from build123d import *

# Parameters (mm, degrees)
BOSS_EXTRUDE1_DEPTH = 390.3
BOSS_EXTRUDE2_DEPTH = 4.3
SKETCH3_W           = 8.6
SKETCH3_H           = 70
CUT_EXTRUDE1_DEPTH  = 10
SKETCH4_W           = 230.803227125
SKETCH4_H           = 349.257793427
CUT_EXTRUDE2_DEPTH  = 15


with BuildPart() as part:
    # Sketch1 → Boss-Extrude1 (new body)
    with BuildSketch(Plane.XY):
        Polygon((-30, 0), (-25.7, 0), (-25.7, 20.7), (25.7, 20.7), (25.7, 0), (30, 0), (30, 25), (-30, 25), align=None)
    extrude(amount=BOSS_EXTRUDE1_DEPTH)

    # Sketch2 → Boss-Extrude2 (add)
    with BuildSketch(Plane(origin=(30, 0, 0), x_dir=(0, 0, -1), z_dir=(1, 0, 0))):
        Polygon((-306, -12.31), (0, 0), (-390.3, 0), (-390.3, -12.31), align=None)
    boss_extrude2 = extrude(amount=-BOSS_EXTRUDE2_DEPTH)

    # Mirror1: Boss-Extrude2 across plane
    add(boss_extrude2.mirror(Plane(origin=(0, 0, 0), x_dir=(0, 0, 1), z_dir=(1, 0, 0))))

    # Sketch3 → Cut-Extrude1 (cut)
    with BuildSketch(Plane(origin=(0, 25, 0), x_dir=(1, 0, 0), z_dir=(0, 1, 0))):
        with Locations((0, -35)):
            Rectangle(SKETCH3_W, SKETCH3_H)
    extrude(amount=-CUT_EXTRUDE1_DEPTH, mode=Mode.SUBTRACT)

    # Sketch4 → Cut-Extrude2 (cut)
    with BuildSketch(Plane(origin=(0, 25, 0), x_dir=(1, 0, 0), z_dir=(0, 1, 0))):
        with Locations((42.992725749, -131.371103286)):
            Rectangle(SKETCH4_W, SKETCH4_H)
    extrude(amount=-CUT_EXTRUDE2_DEPTH, mode=Mode.SUBTRACT)


solid = part.part
Verification items for the finished model (mm, model axes). A direction names the side the tool comes from. Coordinates: 2 decimals unless noted, no trailing zeros. Write each loop counter-clockwise with the first axis right and the second up, starting at its lowest first coordinate (ties: lowest second). Pieces come first, ordered by that corner, then holes. Notation, with made-up numbers: M 46.5,46 L 76.5,46 A33 ccw 76.5,78 Z; hole C -29,6 d9. An arc over 180 degrees is marked long. Use CSV: the item, a comma, the result in double quotes.
Q1. Go/stop test with flat-tipped pins: P1, Ø12, axis at x = -10.5, y = 20.5, coming from the -Z side; P2, Ø12, axis at x = 19.5, z = 325, coming from the -Y side; P3, Ø6, axis at y = 12.5, z = 133, coming from the +X side; P4, Ø4.5, axis at x = -29, z = 114, coming from the +Y side. Record where each tip stops, or that it passes through.
Computed values:
P1,"z = 306"
P2,"y = 20.7"
P3,"x = 30"
P4,"y = 10"
Q2. Section check B-B, the plane z = 166. Enter the section's corners in (x, y).
Computed values:
outline,"M -30,-6.68 L -25.7,-6.68 L -25.7,10 L -30,10 Z; M 25.7,-6.68 L 30,-6.68 L 30,10 L 25.7,10 Z"
Q3. Set-up check for faces 5 (the flat face through (0, 20.7, 348)), 6 (the flat face through (27.88, -6.24, 155.14)), 7 (the flat face through (0, 21, 306)): record each of +Z, -Z, +X, -X, +Y, -Y from which the full face is reachable in a straight line by a thin tool's end or side.
Computed values:
face 5,"+Z, -Z, -Y"
face 6,"-Z, +X, -X, -Y"
face 7,"-Z, +X, -X, +Y"
Q4. Thickness scan on line 1 along X through (y, z) = (0.5, 172); line 2 along Y through (x, z) = (-6, 314). Record the ranges inside material, lowest first. Write a range as [from, to].
Computed values:
line 1,"[-30, -25.7], [25.7, 30]"
line 2,"[20.7, 25]"
Q5. Section check A-A, the plane y = 16. Enter the section's corners in (x, z).
Computed values:
outline,"M -30,306 L -25.7,306 L -25.7,390.3 L -30,390.3 Z; M 25.7,306 L 30,306 L 30,390.3 L 25.7,390.3 Z"
Q6. Section check C-C, the plane x = 22. Enter the section's corners in (y, z), and give its area (3 significant figures).
Computed values:
outline,"M 20.7,306 L 25,306 L 25,390.3 L 20.7,390.3 Z"
area,"362 mm²"
Q7. Mould release check, pull along X, two halves, no side actions. Record for faces 1 (the flat face through (25.7, 4, 241)), 2 (the flat face through (-27.88, -6.24, 155.14)), 3 (the flat face through (-25.7, 4, 241)), 4 (the flat face through (30, 2, 241)): pulls with the +X half, pulls with the -X half, needs draft (parallel to the pull), parting line crosses it, or undercut.
Computed values:
face 1,"undercut"
face 2,"needs draft"
face 3,"undercut"
face 4,"pulls with the +X half"
